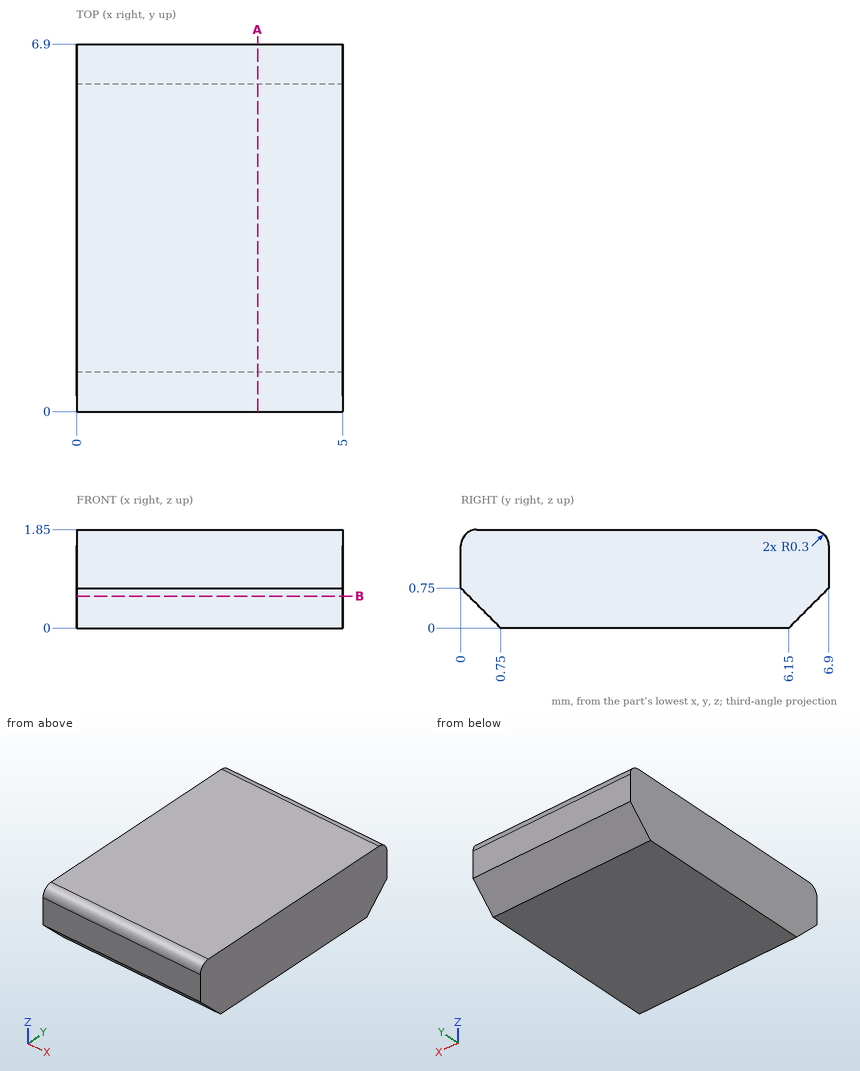
Source: three-view drawing plus pictorial views. Frame: mm from the lowest corner of the part. Round coordinates to 2 decimals unless told otherwise and drop trailing zeros. Loops run counter-clockwise (first coordinate to the right, second up) from the corner with the lowest first, then second, coordinate; pieces in that order, holes last.
1. Ray query, L1, parallel to Y at x = 2.85, z = 0.25; L2, parallel to Y at x = 1.1, z = 0.45. Return the intervals inside material, ascending.
2. Contact query for a flat-ended pin moving along its axis: pin 1 (1.5 mm diameter, centred on x = 1.5, y = 5.5, fed in from -Z). Output: stop coordinate, or through.
3. Section query B-B on z = 0.6. Output: boundary loops of the cut face in (x, y).
4. Section query A-A on x = 3.4. Output: boundary loops of the cut face in (y, z).
Answers below:
1. L1: y = 0.5 to 6.4
1. L2: y = 0.3 to 6.6
2. pin 1: stops at z = 0
3. outline: (0, 0.15) - (5, 0.15) - (5, 6.75) - (0, 6.75) - close
4. outline: (0, 0.75) - (0.75, 0) - (6.15, 0) - (6.9, 0.75) - (6.9, 1.55) arc R0.3 ccw to (6.6, 1.85) - (0.3, 1.85) arc R0.3 ccw to (0, 1.55) - close
